from build123d import *

# Parameters (mm, degrees)
SKETCH1_R                          = 18.05
BOSS_EXTRUDE1_DEPTH                = 41.275
SKETCH6_W                          = 63.5
SKETCH6_H                          = 38.1
CUT_EXTRUDE1_DEPTH                 = 8.89
BOSS_EXTRUDE2_REACH                = 65.289
SKETCH12_W                         = 44
SKETCH12_H                         = 12.7
SKETCH7_W                          = 21.59
SKETCH7_H                          = 82.55
CUT_EXTRUDE2_DEPTH                 = 35
FILLET1_R                          = 10.795
F_1_4_20_TAPPED_HOLE1_AT_2_COUNT   = 2
F_1_4_20_TAPPED_HOLE1_AT_2_PITCH   = 17.986121321
F_1_4_20_TAPPED_HOLE1_AT_3_COUNT   = 2
F_1_4_20_TAPPED_HOLE1_AT_3_PITCH   = 33.234018716
F_1_4_20_TAPPED_HOLE1_AT_4_COUNT   = 2
F_1_4_20_TAPPED_HOLE1_AT_4_PITCH   = 47
F_1_4_20_TAPPED_HOLE1_AT_5_COUNT   = 2
F_1_4_20_TAPPED_HOLE1_AT_5_PITCH   = 43.422338028
F_1_4_20_TAPPED_HOLE1_AT_6_COUNT   = 2
F_1_4_20_TAPPED_HOLE1_AT_6_PITCH   = 33.234018716
F_5_16_18_TAPPED_HOLE1_D           = 6.5278
F_5_16_18_TAPPED_HOLE1_DEPTH       = 20.32
F_5_16_18_TAPPED_HOLE1_CSINK_D     = 9.2075
F_5_16_18_TAPPED_HOLE1_CSINK_ANGLE = 90
F_5_16_18_TAPPED_HOLE1_TIP         = 1.961148974


with BuildPart() as part:
    # Sketch1 → Boss-Extrude1 (new, symmetric)
    with BuildSketch(Plane.XY):
        Polygon((-20.784609691, 22), (20.784609691, 22), (31.75, 3.00738686), (31.75, -22.86), (-31.75, -22.86), (-31.75, 3.00738686), align=None)
        Circle(SKETCH1_R, mode=Mode.SUBTRACT)
    extrude(amount=BOSS_EXTRUDE1_DEPTH, both=True)

    # Sketch6 → Cut-Extrude1 (cut)
    with BuildSketch(Plane.XZ.offset(22.86)):
        Rectangle(SKETCH6_W, SKETCH6_H)
    extrude(amount=-CUT_EXTRUDE1_DEPTH, mode=Mode.SUBTRACT)

    # Sketch12 → Boss-Extrude2 (add, up to next)
    with BuildSketch(Plane.XZ.offset(13.97), mode=Mode.PRIVATE) as boss_extrude2_sk1:
        Rectangle(SKETCH12_W, SKETCH12_H)
    boss_extrude2_tool1 = extrude(boss_extrude2_sk1.sketch, amount=-BOSS_EXTRUDE2_REACH, mode=Mode.PRIVATE) - part.part
    add(boss_extrude2_tool1.solids().sort_by_distance((0, -13.97, 0))[0])

    # Sketch7 → Cut-Extrude2 (cut)
    with BuildSketch(Plane.XZ.offset(22.86)):
        Rectangle(SKETCH7_W, SKETCH7_H)
    extrude(amount=-CUT_EXTRUDE2_DEPTH, mode=Mode.SUBTRACT)

    # Fillet1
    fillet1_edges = [part.edges().sort_by_distance(p)[0] for p in [
        (10.795, 12.14, 0),
        (-10.795, 12.14, 0),
    ]]
    fillet(fillet1_edges, radius=FILLET1_R - 0.0001)  # a hair under: the kernel refuses the full size

    # Sketch3 → 1/4-20 Tapped Hole1 (revolve, cut)
    with BuildSketch(Plane(origin=(-16.617009358, 16.617009358, 41.275), x_dir=(0, -1, 0), z_dir=(1, 0, 0))):
        Polygon((0, 0), (0, 18.043816902), (2.5527, 16.51), (2.5527, 0.635), (3.1877, 0), align=None)
    f_1_4_20_tapped_hole1 = revolve(axis=Axis((-16.617009358, 16.617009358, 47.625), (0, 0, -1)), mode=Mode.SUBTRACT)

    # 1/4-20 Tapped Hole1 at 2: 1/4-20 Tapped Hole1 ×2
    with Locations(*[Vector(-0.38268343236508695, -0.923879532511288, 0) * (i * F_1_4_20_TAPPED_HOLE1_AT_2_PITCH) for i in range(1, F_1_4_20_TAPPED_HOLE1_AT_2_COUNT)]):
        add(f_1_4_20_tapped_hole1, mode=Mode.SUBTRACT)

    # 1/4-20 Tapped Hole1 at 3: 1/4-20 Tapped Hole1 ×2
    with Locations(*[(0, -i * F_1_4_20_TAPPED_HOLE1_AT_3_PITCH, 0) for i in range(1, F_1_4_20_TAPPED_HOLE1_AT_3_COUNT)]):
        add(f_1_4_20_tapped_hole1, mode=Mode.SUBTRACT)

    # 1/4-20 Tapped Hole1 at 4: 1/4-20 Tapped Hole1 ×2
    with Locations(*[Vector(0.7071067811865517, -0.7071067811865434, 0) * (i * F_1_4_20_TAPPED_HOLE1_AT_4_PITCH) for i in range(1, F_1_4_20_TAPPED_HOLE1_AT_4_COUNT)]):
        add(f_1_4_20_tapped_hole1, mode=Mode.SUBTRACT)

    # 1/4-20 Tapped Hole1 at 5: 1/4-20 Tapped Hole1 ×2
    with Locations(*[Vector(0.9238795325112865, -0.38268343236509034, 0) * (i * F_1_4_20_TAPPED_HOLE1_AT_5_PITCH) for i in range(1, F_1_4_20_TAPPED_HOLE1_AT_5_COUNT)]):
        add(f_1_4_20_tapped_hole1, mode=Mode.SUBTRACT)

    # 1/4-20 Tapped Hole1 at 6: 1/4-20 Tapped Hole1 ×2
    with Locations(*[(i * F_1_4_20_TAPPED_HOLE1_AT_6_PITCH, 0, 0) for i in range(1, F_1_4_20_TAPPED_HOLE1_AT_6_COUNT)]):
        add(f_1_4_20_tapped_hole1, mode=Mode.SUBTRACT)

    # Mirror1: 1/4-20 Tapped Hole1 across plane
    add(f_1_4_20_tapped_hole1.mirror(Plane.XY), mode=Mode.SUBTRACT)

    # Mirror1 copy 1 sketch → Mirror1 copy 1 (revolve, cut)
    with BuildSketch(Plane(origin=(-23.5, 0, -41.275), x_dir=(0, -1, 0), z_dir=(1, 0, 0))):
        Polygon((0, 0), (0, -18.043816902), (2.5527, -16.51), (2.5527, -0.635), (3.1877, 0), align=None)
    revolve(axis=Axis((-23.5, 0, -47.625), (0, 0, -1)), mode=Mode.SUBTRACT)

    # Mirror1 copy 2 sketch → Mirror1 copy 2 (revolve, cut)
    with BuildSketch(Plane(origin=(-16.617009358, -16.617009358, -41.275), x_dir=(0, -1, 0), z_dir=(1, 0, 0))):
        Polygon((0, 0), (0, -18.043816902), (2.5527, -16.51), (2.5527, -0.635), (3.1877, 0), align=None)
    revolve(axis=Axis((-16.617009358, -16.617009358, -47.625), (0, 0, -1)), mode=Mode.SUBTRACT)

    # Mirror1 copy 3 sketch → Mirror1 copy 3 (revolve, cut)
    with BuildSketch(Plane(origin=(16.617009358, -16.617009358, -41.275), x_dir=(0, -1, 0), z_dir=(1, 0, 0))):
        Polygon((0, 0), (0, -18.043816902), (2.5527, -16.51), (2.5527, -0.635), (3.1877, 0), align=None)
    revolve(axis=Axis((16.617009358, -16.617009358, -47.625), (0, 0, -1)), mode=Mode.SUBTRACT)

    # Mirror1 copy 4 sketch → Mirror1 copy 4 (revolve, cut)
    with BuildSketch(Plane(origin=(23.5, 0, -41.275), x_dir=(0, -1, 0), z_dir=(1, 0, 0))):
        Polygon((0, 0), (0, -18.043816902), (2.5527, -16.51), (2.5527, -0.635), (3.1877, 0), align=None)
    revolve(axis=Axis((23.5, 0, -47.625), (0, 0, -1)), mode=Mode.SUBTRACT)

    # Mirror1 copy 5 sketch → Mirror1 copy 5 (revolve, cut)
    with BuildSketch(Plane(origin=(16.617009358, 16.617009358, -41.275), x_dir=(0, -1, 0), z_dir=(1, 0, 0))):
        Polygon((0, 0), (0, -18.043816902), (2.5527, -16.51), (2.5527, -0.635), (3.1877, 0), align=None)
    revolve(axis=Axis((16.617009358, 16.617009358, -47.625), (0, 0, -1)), mode=Mode.SUBTRACT)

    # 5/16-18 Tapped Hole1
    with Locations(Plane(origin=(0, -13.97, 0), x_dir=(-1, 0, 0), z_dir=(0, -1, 0))):
        with Locations((-25.4, 0), (25.4, 0)):
            CounterSinkHole(F_5_16_18_TAPPED_HOLE1_D / 2, F_5_16_18_TAPPED_HOLE1_CSINK_D / 2, depth=F_5_16_18_TAPPED_HOLE1_DEPTH, counter_sink_angle=F_5_16_18_TAPPED_HOLE1_CSINK_ANGLE)
            with Locations((0, 0, -(F_5_16_18_TAPPED_HOLE1_DEPTH + F_5_16_18_TAPPED_HOLE1_TIP / 2))):  # 118° drill point
                Cone(0, F_5_16_18_TAPPED_HOLE1_D / 2, F_5_16_18_TAPPED_HOLE1_TIP, mode=Mode.SUBTRACT)


solid = part.part
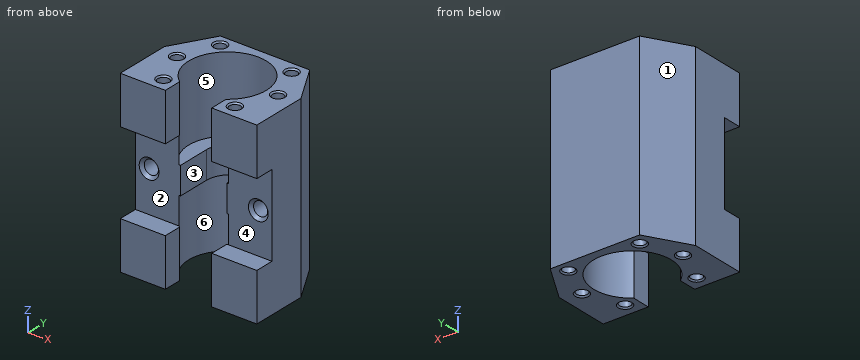
Geometry check sheet. Reference: the model listing, model coordinates, mm. Face numbers are marked on the shaded views. A direction names the side the tool comes from. Round coordinates to 2 decimals unless told otherwise and drop trailing zeros. Order: outer loops, then holes, each group sorted by start corner. A loop starts at its lowest first (then second) coordinate and runs counter-clockwise, first axis right, second up. Notation, with made-up numbers: M 49,25 L 92,25 A33 ccw 92,54 Z; hole C -5,45.5 d3. An arc over 180 degrees is marked long. Write each question's results on one line, items separated by ' | '. Start each with the question number.
1. Cross-section at B-B on x = -1. Record the boundary of the cut face in (y, z) (3 decimals), plus the area to 3 significant figures.
2. Cross-section at A-A on z = 30. Record the boundary of the cut face in (x, y) (3 decimals).
3. Draft check along X on the marked faces 1, 2 and 3. Enter one of: pulls with the +X half, pulls with the -X half, needs draft (parallel to the pull), parting line crosses it, or undercut.
4. Go/stop test with flat-tipped pins: P1, Ø3, axis at x = -16.62, y = -16.62, coming from the -Z side (3 decimals); P2, Ø4, axis at x = 16.62, y = 16.62, coming from the -Z side; P3, Ø6, axis at x = 16.62, y = -16.62, coming from the +Z side. Record where each tip stops, or that it passes through.
5. Material ranges on L1, parallel to X at y = 0, z = -31; L2, parallel to Z at x = -25.4, y = -3.75 (3 decimals); L3, parallel to Z at x = 27.5, y = -20 (3 decimals), recorded low to high. Write a range as from..to.
6. Set-up check for the marked faces 4, 5 and 6: record each of +Z, -Z, +X, -X, +Y, -Y from which the full face is reachable in a straight line by a thin tool's end or side.
7. Cross-section at C-C on z = 10.5. Record the boundary of the cut face in (x, y), plus the area to 3 significant figures.
Resolved:
1) outline: M 12.094,-6.35 L 18.022,-6.35 L 18.022,-41.275 L 22,-41.275 L 22,41.275 L 18.022,41.275 L 18.022,6.35 L 12.094,6.35 Z | area: 404 mm2
2) outline: M -31.75,-22.86 L -10.795,-22.86 L -10.795,-14.466 A18.05 cw long 10.795,-14.466 L 10.795,-22.86 L 31.75,-22.86 L 31.75,3.007 L 20.785,22 L -20.785,22 L -31.75,3.007 Z; hole C -23.5,0 d5.105; hole C -16.617,-16.617 d5.105; hole C -16.617,16.617 d5.105; hole C 16.617,-16.617 d5.105; hole C 16.617,16.617 d5.105; hole C 23.5,0 d5.105
3) face 1: pulls with the -X half | face 2: needs draft | face 3: undercut
4) P1: z = -24.135 | P2: z = -24.44 | P3: z = 41.09
5) L1: -31.75..-26.05, -20.95..-18.05, 18.05..20.95, 26.05..31.75 | L2: -41.275..-3.264, 3.264..41.275 | L3: -41.275..-19.05, 19.05..41.275
6) face 4: +X, -X, -Y | face 5: +Z | face 6: -Z
7) outline: M -31.75,-13.97 L -11.43,-13.97 A18.05 cw long 11.43,-13.97 L 31.75,-13.97 L 31.75,3.01 L 20.78,22 L -20.78,22 L -31.75,3.01 Z | area: 1,120 mm2
